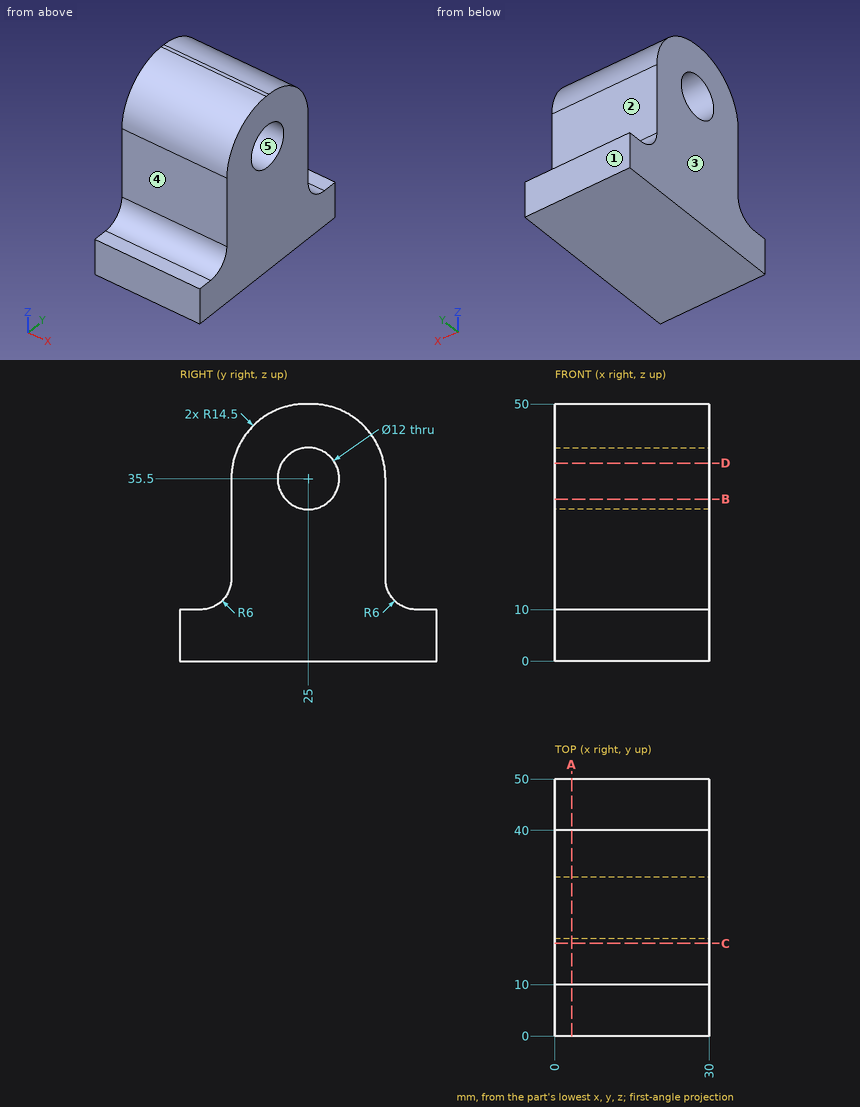
For this review, use the dimensioned drawing (mm, ordinates from the lowest corner) and the shaded views. A direction names the side the tool comes from. Give positions to 0.01 mm unless a question says otherwise; leave off trailing zeros. Write each loop counter-clockwise with the first axis right and the second up, starting at its lowest first coordinate (ties: lowest second). Pieces come first, ordered by that corner, then holes. Notation, with made-up numbers: M 35.25,17 L 39.25,17 A22 ccw 39.25,32 Z; hole C 22,-39 d6. An arc over 180 degrees is marked long. Answer as a JSON object with one key per item and string values. Group by question number.
Item 1: Consider section B-B on z = 31.5. Write out the cut boundary in (x, y).
Item 2: Consider section C-C on y = 18. Write out the cut boundary in (x, z), plus the area to 3 significant figures.
Item 3: Consider section D-D on z = 38.5. Write out the cut boundary in (x, y), plus the area to 3 significant figures.
Item 4: Consider section A-A on x = 3.25. Write out the cut boundary in (y, z).
Item 5: For pin 1 Ø1.5 at (x, z) = (11.5, 29) entering from +Y; pin 2 Ø6 at (x, z) = (19.5, 22) entering from -Y; pin 3 Ø1.5 at (x, y) = (26.5, 29.5) entering from +Z, all flat-tipped, find the tip position at first contact; note any pin that passes through.
Item 6: Tool access review of the marked faces 1 and 2: name each direction out of +Z, -Z, +X, -X, +Y, -Y from which nothing blocks a thin tool from reaching the whole face with its end or side.
Item 7: Draft analysis for pull direction Y (two halves, no side actions). For the marked faces 3, 4 and 5, state which applies: +Y half, -Y half, draft (parallel to the pull), parting line (faces both ways), or undercut.
Item 8: For probe 1 along Y at (x, z) = (16.5, 35.5); probe 2 along Z at (x, y) = (10.75, 4); probe 3 along Y at (x, z) = (24.25, 25), list the stretches that pass through material, from the lowest coordinate up. Write a range as [from, to].
Check result:
{
 "1": {"outline": "M 0,10 L 30,10 L 30,20.53 L 0,20.53 Z; M 0,29.47 L 30,29.47 L 30,40 L 0,40 Z"},
 "2": {"outline": "M 0,0 L 30,0 L 30,48.46 L 0,48.46 Z", "area": "1,450 mm^2"},
 "3": {"outline": "M 0,10.31 L 30,10.31 L 30,19.8 L 0,19.8 Z; M 0,30.2 L 30,30.2 L 30,39.69 L 0,39.69 Z", "area": "569 mm^2"},
 "4": {"outline": "M 0,0 L 50,0 L 50,10 L 46,10 A6 cw 40,16 L 40,35.5 A14.5 ccw 25.5,50 L 24.5,50 A14.5 ccw 10,35.5 L 10,16 A6 cw 4,10 L 0,10 Z; hole C 25,35.5 d12"},
 "5": {"pin 1": "stops at y = 40", "pin 2": "stops at y = 10", "pin 3": "stops at z = 49.63"},
 "6": {"face 1": "+Z, -Z, +X, -X, +Y", "face 2": "+Z, +X, -X, +Y"},
 "7": {"face 3": "draft", "face 4": "-Y half", "face 5": "undercut"},
 "8": {"probe 1": "y = [10, 19], [31, 40]", "probe 2": "z = [0, 10]", "probe 3": "y = [10, 40]"}
}
